from build123d import *

# Parameters (mm, degrees)
SKETCH_1_R          = 1.5
EXTRUDE_1_DEPTH     = 2
EXTRUDE_START       = -2
EXTRUDE_2_DEPTH     = 2
CUT_EXTRUDE_6_DEPTH = 10
EXTRUDE_3_DEPTH     = 2


with BuildPart() as part:
    # 草图1 → 凸台-拉伸1 (new body)
    with BuildSketch(Plane.XY):
        with BuildLine():
            add(Edge.make_bspline(
                [(-7.987888182, 5.955967098), (-3.743831448, 6.072814335), (1.964500208, 2.606366835), (9.971098404, -1.64370968), (11.281519782, -4.915475191), (12.099924554, -5.060596909)],
                knots=[0, 0, 0, 0, 0.492049643, 0.9167731, 1, 1, 1, 1], degree=3))
            ThreePointArc((-7.987888182, 5.955967098), (-11.335902649, 3.978599082), (-9.919857427, 0.35727321))
            add(Edge.make_bspline(
                [(-9.919857427, 0.35727321), (-6.214513301, -1.633496474), (-3.207757144, -4.777239805), (7.078147627, -11.27345607), (9.126976019, -10.694820948), (11.080759462, -10.970561794)],
                knots=[0, 0, 0, 0, 0.359134016, 0.783116461, 1, 1, 1, 1], degree=3))
            ThreePointArc((11.080759462, -10.970561794), (14.456363123, -8.509820643), (12.099924554, -5.060596909))
        make_face()
        with BuildLine():
            ThreePointArc((-1.266260939, -0.840822951), (-0.840822951, 1.266260939), (1.266260939, 0.840822951))
            add(Edge.make_bspline(
                [(1.266260939, 0.840822951), (1.572421217, 0.37975228), (2.2006023, -0.51199535), (3.651531179, -2.318328255), (5.731244794, -4.36936802), (8.515750536, -6.078268968), (10.483635949, -6.491801521), (11.482195768, -6.480104277)],
                knots=[0, 0, 0, 0, 0.125, 0.25, 0.5, 0.75, 1, 1, 1, 1], degree=3))
            ThreePointArc((11.482195768, -6.480104277), (12.568489019, -6.918921272), (13.02, -8))
            ThreePointArc((13.02, -8), (12.581078728, -9.068489019), (11.517804232, -9.519895723))
            add(Edge.make_bspline(
                [(-1.266260939, -0.840822951), (-0.926702959, -1.352189828), (-0.233155533, -2.337077502), (1.395542848, -4.364895632), (3.78940322, -6.741408475), (6.71258634, -8.559402396), (9.358185118, -9.384824122), (10.805124931, -9.52824413), (11.517804232, -9.519895723)],
                knots=[0, 0, 0, 0, 0.125, 0.25, 0.5, 0.75, 0.875, 1, 1, 1, 1], degree=3))
        make_face(mode=Mode.SUBTRACT)
        with Locations((-8.5, 3)):
            Circle(SKETCH_1_R, mode=Mode.SUBTRACT)
    extrude(amount=EXTRUDE_1_DEPTH)

    # 草图2 → 凸台-拉伸2 (add)
    with BuildSketch(Plane.XY.offset(2).offset(EXTRUDE_START)):
        with BuildLine():
            ThreePointArc((12.382013346, -5.132587847), (12.241842746, -5.093168505), (12.099924554, -5.060596909))
            add(Edge.make_bspline(
                [(12.099924554, -5.060596909), (11.281519782, -4.915475191), (10.976298239, -4.153420073), (10.521531787, -3.451743028), (10.374807656, -3.248589277)],
                knots=[0, 0, 0, 0, 0.0832269, 0.118311098, 0.118311098, 0.118311098, 0.118311098], degree=3))
            add(Edge.make_bspline(
                [(10.374807656, -3.248589277), (10.663783201, -3.648703868), (11.898898367, -4.983982122), (12.382013346, -5.132587847)],
                knots=[0, 0, 0, 0, 1, 1, 1, 1], degree=3))
        make_face()
    extrude(amount=EXTRUDE_2_DEPTH)

    # 草图7 → 切除-拉伸6 (cut)
    with BuildSketch(Plane.XY.offset(2)):
        with BuildLine():
            Line((-7.987888182, 5.955967098), (1.266062019, 11.163030358))
            Line((1.266062019, 11.163030358), (12.382013346, -5.132587847))
            add(Edge.make_bspline(
                [(-7.987888182, 5.955967098), (-0.077844738, 4.310798263), (5.452050398, -1.616496795), (12.382013346, -5.132587847)],
                knots=[0, 0, 0, 0, 1, 1, 1, 1], degree=3))
        make_face()
    extrude(amount=-CUT_EXTRUDE_6_DEPTH, mode=Mode.SUBTRACT)

    # 草图8 → 凸台-拉伸3 (add)
    with BuildSketch(Plane.XY.offset(2).offset(EXTRUDE_START)):
        with BuildLine():
            ThreePointArc((14.472568825, -7.595235155), (13.787052442, -6.058508015), (12.382013346, -5.132587847))
            add(Edge.make_bspline(
                [(12.382013346, -5.132587847), (12.317985887, -5.112893059), (12.24075005, -5.072355166), (12.154258782, -5.015913393)],
                knots=[0, 0, 0, 0, 0.132530478, 0.132530478, 0.132530478, 0.132530478], degree=3))
            add(Edge.make_bspline(
                [(12.154258782, -5.015913393), (8.423758186, -3.086650873), (5.090409864, -0.473998081), (1.556721967, 1.76411334)],
                knots=[0, 0, 0, 0, 0.540677693, 0.540677693, 0.540677693, 0.540677693], degree=3))
            add(Edge.make_bspline(
                [(1.556721967, 1.76411334), (4.495628992, -0.097285168), (12.132556571, -1.344060553), (14.312894291, -6.422594924), (14.472568825, -7.595235155)],
                knots=[0, 0, 0, 0, 0.805722027, 1, 1, 1, 1], degree=3))
        make_face()
    extrude(amount=EXTRUDE_3_DEPTH)


solid = part.part
Input: part model. Units: mm. Frame: model coordinates. Coordinates: 2 decimals unless noted, no trailing zeros. Answer in a Markdown table with one row per item.
(1) Material intervals for line 1 (Y direction, x = 6.25, z = 1.5); line 2 (X direction, y = -8.5, z = 0.95); line 3 (X direction, y = 3.75, z = 1.35), sorted ascending. Write a range as [from, to].
Numbers:
| item | result |
|---|---|
| line 1 | y = [-10.2, -8.18], [-4.6, -0.29] |
| line 2 | x = [2.94, 6.91], [12.94, 14.46] |
| line 3 | x = [-11.4, -9.8], [-7.2, -1.89] |
(2) Section query A-A, the plane z = 1.65. Give the number of separate pieces and of enclosed holes in the cut face, plus the area to 3 significant figures.
Numbers:
| item | result |
|---|---|
| separate pieces | 1 |
| enclosed holes | 2 |
| area | 151 mm^2 |
(3) Contact query for flat-ended pins moving along their axis: pin 1 Ø3 at (x, y) = (7, -7.5) entering from +Z; pin 2 Ø1.8 at (x, y) = (-8.5, 3) entering from +Z. Output: stop coordinate, or through.
Numbers:
| item | result |
|---|---|
| pin 1 | stops at z = 2 |
| pin 2 | passes through |
(4) Draft query along Y for faces 1 (the flat face through (0, -3, 0)), 2 (the cylindrical face through (-9.7, 2.1, 1)), 3 (the cylindrical face through (-0.868, 1.247, 0.986)), 4 (the cylindrical face through (-11.316, 4.034, 0.986)). Return one class per face: pulls with the +Y half, pulls with the -Y half, needs draft (parallel to the pull), parting line crosses it, or undercut.
Numbers:
| item | result |
|---|---|
| face 1 | needs draft |
| face 2 | undercut |
| face 3 | undercut |
| face 4 | parting line crosses it |
